Check sheet for the modelled part. Datum: model origin and axes. Units: mm. Face numbers are marked on the shaded views. A direction names the side the tool comes from. Coordinates: 2 decimals unless noted, no trailing zeros. Loops run counter-clockwise (first coordinate to the right, second up) from the corner with the lowest first, then second, coordinate; pieces in that order, holes last.
```python
from build123d import *

# Parameters (mm, degrees)
SKETCH1_W               = 8
SKETCH1_H               = 8
BOSS_EXTRUDE1_DEPTH     = 3
CUT_EXTRUDE1_DEPTH      = 12.704699911
CUT_EXTRUDE1_DEPTH_BACK = 12.704699911
CUT_EXTRUDE2_DEPTH      = 11
SKETCH4_R               = 1.8
CUT_EXTRUDE3_DEPTH      = 0.8
SKETCH5_W               = 8
SKETCH5_H               = 1
BOSS_EXTRUDE2_DEPTH     = 2
FILLET1_R               = 4
CUT_EXTRUDE4_DEPTH      = 0.4


with BuildPart() as part:
    # Sketch1 → Boss-Extrude1 (new body)
    with BuildSketch(Plane(origin=(0, 0, 0), x_dir=(1, 0, 0), z_dir=(0, 1, 0))):
        with Locations((4, 4)):
            Rectangle(SKETCH1_W, SKETCH1_H)
    extrude(amount=BOSS_EXTRUDE1_DEPTH)

    # Sketch2 → Cut-Extrude1 (cut, two sides: drawn at the far end of the back side and taken through both)
    with BuildSketch(Plane.XY.offset(-CUT_EXTRUDE1_DEPTH_BACK)):
        Polygon((0, 0), (0.6, 3), (0, 3), align=None)
        Polygon((8, 0), (7.4, 3), (8, 3), align=None)
    extrude(amount=CUT_EXTRUDE1_DEPTH + CUT_EXTRUDE1_DEPTH_BACK, mode=Mode.SUBTRACT)

    # Sketch3 → Cut-Extrude2 (cut)
    with BuildSketch(Plane(origin=(0, 0, 0), x_dir=(0, 0, -1), z_dir=(1, 0, 0))):
        Polygon((0, 0), (0.6, 3), (0, 3), align=None)
        Polygon((8, 3), (7.4, 3), (8, 0), align=None)
    extrude(amount=CUT_EXTRUDE2_DEPTH, mode=Mode.SUBTRACT)

    # Sketch4 → Cut-Extrude3 (cut)
    with BuildSketch(Plane.XZ):
        with Locations(Location((4, -3.75, 0), (0, 0, 270))):
            Circle(SKETCH4_R)
    extrude(amount=-CUT_EXTRUDE3_DEPTH, mode=Mode.SUBTRACT)

    # Sketch5 → Boss-Extrude2 (add)
    with BuildSketch(Plane.XZ):
        with Locations((4, -7.5)):
            Rectangle(SKETCH5_W, SKETCH5_H)
    extrude(amount=BOSS_EXTRUDE2_DEPTH)

    # Fillet1
    # the kernel refuses this fillet: 4 mm, written as the material it takes off along each edge
    with BuildSketch(Plane(origin=(8, -2, -16.660254038), x_dir=(0, 1, 0), z_dir=(0, 0, 1)), Plane(origin=(0, -2, 1.660254038), x_dir=(0, 1, 0), z_dir=(0, 0, -1))) as fillet1_piece_1:
        with BuildLine():
            CenterArc((4, 3.464101615), FILLET1_R, 180, 60)
            Line((0, 3.464101615), (-0.08, 3.464101615))
            Line((-0.08, 3.464101615), (-0.08, 0))
            Line((-0.08, 0), (0, -0.08))
            ThreePointArc((0, -0.08), (1, -0.08), (1.96, -0.069282032))
            Line((1.96, -0.069282032), (2, 0))
        make_face()
    extrude(amount=18.320508076, mode=Mode.SUBTRACT)

    # Sketch6 → Cut-Extrude4 (cut)
    with BuildSketch(Plane(origin=(0, 3, 0), x_dir=(1, 0, 0), z_dir=(0, 1, 0))):
        with BuildLine():
            Line((4.984953699, 3.505457585), (5.754184468, 3.249047329))
            add(Edge.make_bspline(
                [(5.754184468, 3.249047329), (5.738551331, 3.198610805), (5.707936732, 3.099840225), (5.651723194, 2.958278532), (5.587443886, 2.827086856), (5.517410433, 2.704729688), (5.437267593, 2.594367909), (5.351502188, 2.492347505), (5.25756407, 2.400817223), (5.155916755, 2.319581611), (5.047538657, 2.247743191), (4.931170847, 2.187011676), (4.808549951, 2.134705195), (4.678432524, 2.092325917), (4.541682112, 2.058386549), (4.397657073, 2.035969411), (4.247031142, 2.020769852), (4.144181592, 2.01912185), (4.091524212, 2.018278098)],
                knots=[0, 0, 0, 0, 1.126640671, 2.206316847, 3.246446654, 4.24268115, 5.210795778, 6.153057602, 7.084219323, 8.004711971, 8.926421631, 9.854560063, 10.802134612, 11.768317461, 12.772025444, 13.805668576, 14.876536225, 16, 16, 16, 16], degree=3))
            add(Edge.make_bspline(
                [(4.091524212, 2.018278098), (4.026529436, 2.019622049), (3.898682769, 2.022265641), (3.711719127, 2.048877042), (3.533551231, 2.090397174), (3.363924198, 2.147881075), (3.203970267, 2.224018355), (3.052230113, 2.31567777), (2.909808045, 2.424720155), (2.777203704, 2.549307725), (2.656729454, 2.688489389), (2.552550394, 2.841513049), (2.46353299, 3.006222974), (2.391584534, 3.18340452), (2.335325697, 3.372875751), (2.295916265, 3.574374695), (2.271256348, 3.787964822), (2.268446864, 3.934340923), (2.267004981, 4.009463995)],
                knots=[0, 0, 0, 0, 1.025049111, 2.016302254, 2.973197159, 3.90886983, 4.83646737, 5.763135642, 6.70136783, 7.661478232, 8.629732022, 9.600038443, 10.576877021, 11.5787097, 12.612181225, 13.690866959, 14.814907849, 16, 16, 16, 16], degree=3))
            add(Edge.make_bspline(
                [(2.267004981, 4.009463995), (2.268440364, 4.088592426), (2.271240535, 4.242957555), (2.295946649, 4.467391238), (2.33430142, 4.6789069), (2.390655342, 4.87619306), (2.461546504, 5.060638151), (2.550671985, 5.230411199), (2.653811862, 5.387775744), (2.773739341, 5.529847487), (2.90694801, 5.655987983), (3.049697575, 5.767530284), (3.203319761, 5.861106277), (3.366973913, 5.937627827), (3.540879519, 5.996843969), (3.724694381, 6.039484239), (3.918568892, 6.064303618), (4.051121857, 6.067784001), (4.118767802, 6.069560149)],
                knots=[0, 0, 0, 0, 1.212648312, 2.365655595, 3.457000981, 4.504219827, 5.506356588, 6.480637568, 7.437950897, 8.385265166, 9.323599949, 10.245787653, 11.157260172, 12.074946661, 13.00980897, 13.968233668, 14.963125779, 16, 16, 16, 16], degree=3))
            add(Edge.make_bspline(
                [(4.118767802, 6.069560149), (4.177845619, 6.068071541), (4.293675542, 6.065152928), (4.463296702, 6.045323759), (4.624050093, 6.010524892), (4.776804639, 5.963554159), (4.920690778, 5.901565287), (5.05596628, 5.825815524), (5.18309612, 5.736705664), (5.259694467, 5.667100309), (5.298254981, 5.632060149)],
                knots=[0, 0, 0, 0, 1.098510076, 2.153775193, 3.169777012, 4.153122333, 5.120892526, 6.076995459, 7.031936742, 8, 8, 8, 8], degree=3))
            add(Edge.make_bspline(
                [(5.298254981, 5.632060149), (5.320604149, 5.60976374), (5.365827451, 5.564647194), (5.426213252, 5.488477681), (5.483466493, 5.406481188), (5.536678451, 5.317258958), (5.58416733, 5.220136739), (5.628218337, 5.11660602), (5.668774447, 5.006267724), (5.691328308, 4.929479087), (5.702902417, 4.89007297)],
                knots=[0, 0, 0, 0, 0.885292881, 1.791380647, 2.722937556, 3.69093542, 4.703306561, 5.754477758, 6.847650944, 8, 8, 8, 8], degree=3))
            Line((5.702902417, 4.89007297), (4.933671648, 4.736226816))
            add(Edge.make_bspline(
                [(4.933671648, 4.736226816), (4.927133502, 4.76145763), (4.914255072, 4.811155713), (4.888197319, 4.88256913), (4.858307022, 4.950334085), (4.821260737, 5.012790777), (4.781908002, 5.072717729), (4.735316585, 5.127453998), (4.684461977, 5.178434101), (4.62897783, 5.22512899), (4.569525593, 5.266595122), (4.507249934, 5.303870591), (4.441018967, 5.334299022), (4.371713727, 5.358915551), (4.29961025, 5.379554656), (4.224066596, 5.392304393), (4.145731594, 5.40209207), (4.092359182, 5.40262243), (4.065081904, 5.402893482)],
                knots=[0, 0, 0, 0, 1.051226935, 2.070641259, 3.064374968, 4.034983734, 4.997599858, 5.953980297, 6.92954377, 7.901109626, 8.875958313, 9.851998019, 10.826131395, 11.811470594, 12.818270757, 13.847890818, 14.900111925, 16, 16, 16, 16], degree=3))
            add(Edge.make_bspline(
                [(4.065081904, 5.402893482), (4.027621622, 5.402136956), (3.95451036, 5.400660441), (3.84764705, 5.384198307), (3.745794169, 5.361223694), (3.649362485, 5.32614158), (3.558949174, 5.281271846), (3.473526684, 5.226727667), (3.393563858, 5.162742669), (3.319033671, 5.088558841), (3.252152959, 5.002834902), (3.193355266, 4.905393862), (3.144577309, 4.795129453), (3.104977365, 4.673123713), (3.073807698, 4.539086512), (3.051550102, 4.39284594), (3.039240982, 4.234301954), (3.037259111, 4.124602201), (3.03623575, 4.067957585)],
                knots=[0, 0, 0, 0, 0.938194206, 1.831074359, 2.704771284, 3.551924377, 4.396294915, 5.230222094, 6.087631332, 6.958733431, 7.860107878, 8.806247581, 9.804197948, 10.875520245, 12.017191412, 13.250061517, 14.580040491, 16, 16, 16, 16], degree=3))
            add(Edge.make_bspline(
                [(3.03623575, 4.067957585), (3.037249034, 4.007841988), (3.039201475, 3.892008492), (3.051507983, 3.724929387), (3.073907907, 3.571260811), (3.104663329, 3.430730056), (3.144462832, 3.303423199), (3.1931583, 3.189560541), (3.251047919, 3.089008738), (3.318041624, 3.001834743), (3.3924457, 2.926952551), (3.472244969, 2.862570915), (3.55696863, 2.80752487), (3.647126515, 2.762236533), (3.743061533, 2.72797641), (3.843985242, 2.703130369), (3.950267946, 2.687335345), (4.023091528, 2.685752793), (4.060274212, 2.684944765)],
                knots=[0, 0, 0, 0, 1.475208372, 2.842499301, 4.107722225, 5.282836115, 6.369007568, 7.375918121, 8.315702116, 9.208439171, 10.065831443, 10.90006451, 11.71996243, 12.54067204, 13.369972975, 14.214060185, 15.088124569, 16, 16, 16, 16], degree=3))
            add(Edge.make_bspline(
                [(4.060274212, 2.684944765), (4.087802914, 2.685631562), (4.141934021, 2.686982048), (4.22194397, 2.695553476), (4.298737204, 2.711910812), (4.3726896, 2.733540427), (4.444088489, 2.760679214), (4.511844803, 2.795492821), (4.577291618, 2.835505891), (4.639070965, 2.882398144), (4.6980101, 2.93504365), (4.751766089, 2.995888735), (4.801629231, 3.063471428), (4.846966938, 3.138243387), (4.889294086, 3.219564589), (4.92530624, 3.308702064), (4.958854788, 3.404215308), (4.976102112, 3.471120718), (4.984953699, 3.505457585)],
                knots=[0, 0, 0, 0, 0.980177776, 1.927374078, 2.859849964, 3.771585772, 4.668674471, 5.574490016, 6.479656464, 7.396337719, 8.332153134, 9.288470092, 10.28125149, 11.318486971, 12.398724812, 13.541284404, 14.738150009, 16, 16, 16, 16], degree=3))
        make_face()
    extrude(amount=-CUT_EXTRUDE4_DEPTH, mode=Mode.SUBTRACT)


solid = part.part
```
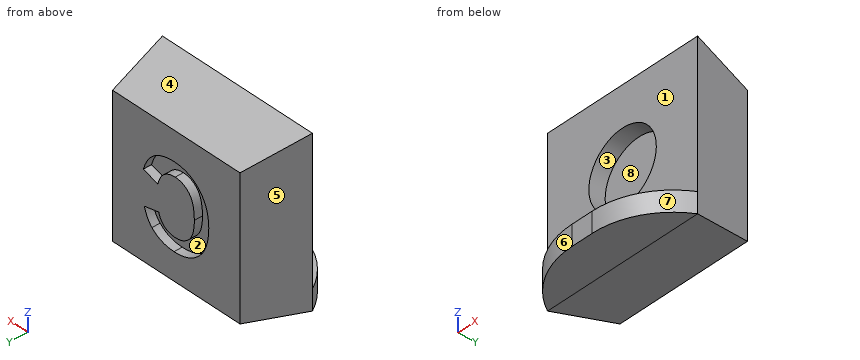
1) Mould release check, pull along X, two halves, no side actions. Record for the marked faces 6, 7 and 8: +X half, -X half, draft (parallel to the pull), parting line (faces both ways), or undercut.
Answer sheet:
face 6: -X half
face 7: +X half
face 8: undercut
2) Section check D-D on y = 1.4. Enter the section's corners in (x, z), plus the area to 3 significant figures.
Answer sheet:
outline: (0.28, -7.72) - (7.72, -7.72) - (7.72, -0.28) - (0.28, -0.28) - close
area: 55.4 mm2
3) Section check C-C on x = 7.5. Enter the section's corners in (y, z).
Answer sheet:
outline: (-0.69, -8) - (0, -8) - (2.5, -7.5) - (2.5, -0.5) - (0, 0) - (0, -7) - (-0.69, -7) - close
4) Section check B-B on z = -6.25. Enter the section's corners in (x, y), plus the area to 3 significant figures.
Answer sheet:
outline: (0, 0) - (8, 0) - (7.4, 3) - (0.6, 3) - close
area: 22.2 mm2
5) Set-up check for the marked faces 1, 2, 3, 4 and 5: record each of +Z, -Z, +X, -X, +Y, -Y from which the full face is reachable in a straight line by a thin tool's end or side.
Answer sheet:
face 1: +Z, +X, -X, -Y
face 2: +Y
face 3: -Y
face 4: +Z, +X, -X, +Y
face 5: +Z, -Z, -X, +Y
6) Depth check by flat-ended pin: pin 1 (1 mm diameter, centred on y = -1, z = -4, fed in from -X); pin 2 (2 mm diameter, centred on x = 1, y = 2, fed in from -Z); pin 3 (3 mm diameter, centred on x = 4, z = -3.75, fed in from -Y); pin 4 (1.6 mm diameter, centred on x = 2, y = -1, fed in from +Z). Enter the tip coordinate at first touch or a pass-through.
Answer sheet:
pin 1: passes through
pin 2: stops at z = -7.8
pin 3: stops at y = 0.8
pin 4: stops at z = -7
7) Section check A-A on y = 0.35. Enter the section's corners in (x, z), plus the area to 3 significant figures.
Answer sheet:
outline: (0.07, -7.93) - (7.93, -7.93) - (7.93, -0.07) - (0.07, -0.07) - close; hole circle Ø3.6 at (4, -3.75)
area: 51.6 mm2
8) Scan lines: line 1 (Y direction, x = 2.5, z = -2.5); line 2 (Y direction, x = 2.5, z = -4.5); line 3 (Z direction, x = 3.25, y = 2.65). Record each from-to range of solid material in increasing order.
Answer sheet:
line 1: y = 0 to 3
line 2: y = 0.8 to 2.6
line 3: z = -7.47 to -5.88, -5 to -3.1, -2.2 to -0.53
